from build123d import *

# Parameters (mm, degrees)
SKETCH1_R           = 22.5
SKETCH1_R_2         = 1.7
SKETCH1_R_3         = 10.5
BOSS_EXTRUDE2_DEPTH = 7
BOSS_EXTRUDE3_START = -1
SKETCH1_3_R         = 24.5
SKETCH1_3_R_2       = 22.5
SKETCH1_3_R_3       = 1.7
SKETCH1_3_R_4       = 10.5
BOSS_EXTRUDE3_DEPTH = 1


with BuildPart() as part:
    # Sketch1 → Boss-Extrude2 (new body)
    with BuildSketch(Plane.XY):
        Circle(SKETCH1_R)
        with Locations((-12.730573436, -7.35)):
            Circle(SKETCH1_R_2, mode=Mode.SUBTRACT)
        with Locations((12.730573436, -7.35)):
            Circle(SKETCH1_R_2, mode=Mode.SUBTRACT)
        with Locations((0, 14.7)):
            Circle(SKETCH1_R_2, mode=Mode.SUBTRACT)
        Circle(SKETCH1_R_3, mode=Mode.SUBTRACT)
    extrude(amount=BOSS_EXTRUDE2_DEPTH)

    # Sketch1_3 → Boss-Extrude3 (add)
    # profile 1 of 2: a face of its own
    with BuildSketch(Plane.XY.offset(BOSS_EXTRUDE3_START)):
        Circle(SKETCH1_3_R)
        Circle(SKETCH1_3_R_2, mode=Mode.SUBTRACT)
    # profile 2 of 2: a face of its own
    with BuildSketch(Plane.XY.offset(BOSS_EXTRUDE3_START)):
        Circle(SKETCH1_3_R_2)
        with Locations((-12.730573436, -7.35)):
            Circle(SKETCH1_3_R_3, mode=Mode.SUBTRACT)
        with Locations((12.730573436, -7.35)):
            Circle(SKETCH1_3_R_3, mode=Mode.SUBTRACT)
        with Locations((0, 14.7)):
            Circle(SKETCH1_3_R_3, mode=Mode.SUBTRACT)
        Circle(SKETCH1_3_R_4, mode=Mode.SUBTRACT)
    extrude(amount=BOSS_EXTRUDE3_DEPTH)


solid = part.part
Source: CAD feature listing. Evaluate the final solid. Frame: model axes, mm. A direction names the side the tool comes from. Coordinates: 2 decimals unless noted, no trailing zeros. Order: outer loops, then holes, each group sorted by start corner. A loop starts at its lowest first (then second) coordinate and runs counter-clockwise, first axis right, second up. Notation, with made-up numbers: M 4,80 L 33,80 A21 cw 33,89 Z; hole C 53.5,28.5 d8. An arc over 180 degrees is marked long. Write each question's results on one line, items separated by ' | '. Start each with the question number.
1. Section A-A, the plane x = 0. Return the cut outline in (y, z).
2. Section B-B, the plane y = 0. Return the cut outline in (x, z).
3. Material intervals for L1, parallel to Y at x = 0, z = 4; L2, parallel to X at y = -7, z = 1; L3, parallel to X at y = 14.5, z = 1.5, sorted ascending.
4. Draft query along X for faces 1 (the face through (11, 0, -1)), 2 (the face through (-0.221, 16.386, 2.944)), 3 (the face through (10.382, -19.961, 3.451)), 4 (the face through (12.36, -9.01, 2.94)). Return one class per face: +X half, -X half, draft (parallel to the pull), parting line (faces both ways), or undercut.
5. Section D-D, the plane z = 5. Return the cut outline in (x, y), then the cut area to 3 significant figures.
6. Reachability of faces 5 (the face through (-11.16, -8, 2.94)), 6 (the face through (11, -20, 0)) from +Z, -Z, +X, -X, +Y, -Y: full face, straight path, thin tool, end or side. Return the list, or none.
7. Pin query (flat end, axial travel): pin 1 (4.5 mm diameter, centred on x = -12.73, y = -7.35, fed in from +Z); pin 2 (2.5 mm diameter, centred on x = 0, y = 14.7, fed in from -Z); pin 3 (1.5 mm diameter, centred on x = 17.5, z = 1.5, fed in from -Y); pin 4 (3 mm diameter, centred on x = -1.5, z = 3, fed in from +Y). Return the tip coordinate at first contact, or that it passes through.
8. Section C-C, the plane x = -8. Return the cut outline in (y, z), then the cut area to 3 significant figures.
Solution:
1) outline: M -24.5,-1 L -10.5,-1 L -10.5,7 L -22.5,7 L -22.5,0 L -24.5,0 Z; M 10.5,-1 L 13,-1 L 13,7 L 10.5,7 Z; M 16.4,-1 L 24.5,-1 L 24.5,0 L 22.5,0 L 22.5,7 L 16.4,7 Z
2) outline: M -24.5,-1 L -10.5,-1 L -10.5,7 L -22.5,7 L -22.5,0 L -24.5,0 Z; M 10.5,-1 L 24.5,-1 L 24.5,0 L 22.5,0 L 22.5,7 L 10.5,7 Z
3) L1: -22.5 to -10.5, 10.5 to 13, 16.4 to 22.5 | L2: -21.38 to -14.39, -11.07 to -7.83, 7.83 to 11.07, 14.39 to 21.38 | L3: -17.2 to -1.69, 1.69 to 17.2
4) face 1: draft | face 2: undercut | face 3: parting line | face 4: undercut
5) outline: C 0,0 d45; hole C -12.73,-7.35 d3.4; hole C 0,0 d21; hole C 0,14.7 d3.4; hole C 12.73,-7.35 d3.4 | area: 1,220 mm²
6) face 5: +Z, -Z | face 6: +Z
7) pin 1: z = 7 | pin 2: through | pin 3: y = -15.02 | pin 4: y = 22.5
8) outline: M -23.16,-1 L -6.8,-1 L -6.8,7 L -21.03,7 L -21.03,0 L -23.16,0 Z; M 6.8,-1 L 23.16,-1 L 23.16,0 L 21.03,0 L 21.03,7 L 6.8,7 Z | area: 232 mm²
